Design review of the part built by this model. Coordinates are the model's own, in mm. A direction names the side the tool comes from. Give positions to 0.01 mm unless a question says otherwise; leave off trailing zeros. Loops run counter-clockwise (first coordinate to the right, second up) from the corner with the lowest first, then second, coordinate; pieces in that order, holes last. Notation, with made-up numbers: (-4.75, -14) -> (54.25, -14) arc R24 ccw to (54.25, 11) -> close; hole circle Ø9 at (38.5, -17). An arc over 180 degrees is marked (long way). Use CSV: the item, a comma, the result in double quotes. Start each with the question number.
Item 1: We need section D-D (x = 12). State the section outline as (y, z) points.
Item 2: The part is to be moulded in two halves that separate along Z. For faces 6 (the face through (0, 8, 55)), 7 (the face through (-5.2, -8, 20)), 8 (the face through (10.944, -6.646, 4.324)), say which applies: +Z half, -Z half, draft (parallel to the pull), parting line (faces both ways), or undercut.
Item 3: Wall thickness on line 1 along Y through (x, z) = (-4.25, 38); line 2 along X through (y, z) = (-3.25, 31.5); line 3 along Z through (x, y) = (-12.75, -4.5): over which ranges is each line inside the solid? List them lowest first. Write a range as from..to.
Item 4: For faces 1 (the face through (0, -8.7, 20)), 2 (the face through (-5, 7, 47)), 3 (the face through (0, 2.5, 47)), 4 (the face through (7, -4, 5)), 5 (the face through (-11.056, -6.646, 5.676)), list the 3-axis set-ups (+Z, -Z, +X, -X, +Y, -Y) from which the entire face can be reached by the end or side of a thin tool; tool diameter is ignored.
Item 5: We need section B-B (x = 2.5). State the section outline as (y, z) points.
Item 6: We need section C-C (y = -4.5). State the section outline as (x, z) points, plus the area to 3 significant figures.
Item 7: Clearance check with a flat-ended pin moving along its axis: pin 1 (3 mm diameter, centred on x = 0, z = 46, fed in from -Y). State where the tip first meets the part, or that it passes through.
from build123d import *

# Parameters (mm, degrees)
ESQUISSE1_W             = 30
ESQUISSE1_H             = 25
BOSS_EXTRU_1_DEPTH      = 40
ENL_V_MAT_EXTRU_1_DEPTH = 45.511234537
ESQUISSE4_R             = 2.25
ENL_V_MAT_EXTRU_2_DEPTH = 8
ENL_V_START             = -8
ESQUISSE5_R             = 2.25
ENL_V_MAT_EXTRU_3_DEPTH = 8
ESQUISSE6_W             = 10
ESQUISSE6_H             = 10
BOSS_EXTRU_2_DEPTH      = 15


with BuildPart() as part:
    # Esquisse1 → Boss.-Extru.1 (new body)
    with BuildSketch(Plane.XY):
        Rectangle(ESQUISSE1_W, ESQUISSE1_H)
    extrude(amount=BOSS_EXTRU_1_DEPTH)

    # Esquisse3 → Enlèv. mat.-Extru.1 (cut, through all)
    with BuildSketch(Plane(origin=(0, 0, 0), x_dir=(-1, 0, 0), z_dir=(0, 0, -1))):
        Polygon((-5.2, 0.7), (-5.2, -3.1), (-4.2, -3.1), (-4.2, -5.9), (-5.2, -5.9), (-5.2, -9.7), (-1.4, -9.7), (-1.4, -8.7), (1.4, -8.7), (1.4, -9.7), (5.2, -9.7), (5.2, -5.9), (4.2, -5.9), (4.2, -3.1), (5.2, -3.1), (5.2, 0.7), (1.4, 0.7), (1.4, -0.3), (-1.4, -0.3), (-1.4, 0.7), align=None)
    extrude(amount=-ENL_V_MAT_EXTRU_1_DEPTH, mode=Mode.SUBTRACT)

    # Esquisse4 → Enlèv. mat.-Extru.2 (cut)
    with BuildSketch(Plane.ZY.offset(15)):
        with Locations(Location((5, -4.5, 0), (0, 0, 270))):
            Circle(ESQUISSE4_R)
    extrude(amount=-ENL_V_MAT_EXTRU_2_DEPTH, mode=Mode.SUBTRACT)

    # Esquisse5 → Enlèv. mat.-Extru.3 (cut)
    with BuildSketch(Plane(origin=(15, 0, 0), x_dir=(0, 0, -1), z_dir=(1, 0, 0)).offset(ENL_V_START)):
        with Locations(Location((-5, -4.5, 0), (0, 0, 270))):
            Circle(ESQUISSE5_R)
    extrude(amount=ENL_V_MAT_EXTRU_3_DEPTH, mode=Mode.SUBTRACT)

    # Esquisse6 → Boss.-Extru.2 (add)
    with BuildSketch(Plane.XY.offset(40)):
        with Locations((0, 7.5)):
            Rectangle(ESQUISSE6_W, ESQUISSE6_H)
    extrude(amount=BOSS_EXTRU_2_DEPTH)


solid = part.part
Results found:
1,outline,"(-12.5, 0) -> (12.5, 0) -> (12.5, 40) -> (-12.5, 40) -> close; hole circle Ø4.5 at (-4.5, 5)"
2,face 6,"+Z half"
2,face 7,"draft"
2,face 8,"undercut"
3,line 1,"-12.5..-9.7, -5.9..-3.1, 0.7..12.5"
3,line 2,"-15..-4.2, 4.2..15"
3,line 3,"0..2.75, 7.25..40"
4,face 1,"+Z, -Z"
4,face 2,"+Z, -X, +Y, -Y"
4,face 3,"+Z, +X, -X, -Y"
4,face 4,"+X"
4,face 5,"-X"
5,outline,"(-12.5, 0) -> (-9.7, 0) -> (-9.7, 40) -> (-12.5, 40) -> close; (0.7, 0) -> (12.5, 0) -> (12.5, 55) -> (2.5, 55) -> (2.5, 40) -> (0.7, 40) -> close"
6,outline,"(-15, 0) -> (-4.2, 0) -> (-4.2, 40) -> (-15, 40) -> (-15, 7.25) -> (-7, 7.25) -> (-7, 2.75) -> (-15, 2.75) -> close; (4.2, 0) -> (15, 0) -> (15, 2.75) -> (7, 2.75) -> (7, 7.25) -> (15, 7.25) -> (15, 40) -> (4.2, 40) -> close"
6,area,"792 mm²"
7,pin 1,"y = 2.5"
